Work out the finished part from the listing and answer in its coordinate system (mm). A direction names the side the tool comes from. Round coordinates to 2 decimals unless told otherwise and drop trailing zeros. Order: outer loops, then holes, each group sorted by start corner. A loop starts at its lowest first (then second) coordinate and runs counter-clockwise, first axis right, second up. Notation, with made-up numbers: (-13, 6) - (0, 6) arc R25 cw to (0, 40) - close; hole circle Ø3 at (-13.75, -10). An arc over 180 degrees is marked (long way). Use CSV: the item, a comma, the result in double quotes.
from build123d import *

# Parameters (mm, degrees)
SKETCH1_R                = 5
BOSS_EXTRUDE1_DEPTH      = 10
SKETCH2_R                = 4.5
BOSS_EXTRUDE2_DEPTH      = 12
BOSS_EXTRUDE2_DEPTH_BACK = 10
SKETCH3_R                = 5
BOSS_EXTRUDE3_DEPTH      = 10
SKETCH4_R                = 6
BOSS_EXTRUDE4_DEPTH      = 2
FILLET1_R                = 3


with BuildPart() as part:
    # Sketch1 → Boss-Extrude1 (new body)
    with BuildSketch(Plane(origin=(0, 0, 0), x_dir=(1, 0, 0), z_dir=(0, 1, 0))):
        with BuildLine():
            ThreePointArc((-10, 0), (0, -10), (10, 0))
            ThreePointArc((10, 0), (-47.75, 57.75), (-105.5, 0))
            ThreePointArc((-105.5, 0), (-95.5, -10), (-85.5, 0))
            ThreePointArc((-85.5, 0), (-47.75, 37.75), (-10, 0))
        make_face()
        with Locations((-95.5, 0)):
            Circle(SKETCH1_R, mode=Mode.SUBTRACT)
        Circle(SKETCH1_R, mode=Mode.SUBTRACT)
    extrude(amount=BOSS_EXTRUDE1_DEPTH)



with BuildPart() as body_2:
    # Sketch2 → Boss-Extrude2 (new body, two sides)
    with BuildSketch(Plane(origin=(0, 10, 0), x_dir=(1, 0, 0), z_dir=(0, 1, 0))) as boss_extrude2_sk:
        Circle(SKETCH2_R)
    extrude(amount=BOSS_EXTRUDE2_DEPTH)
    extrude(boss_extrude2_sk.sketch, amount=-BOSS_EXTRUDE2_DEPTH_BACK)


with BuildPart() as part_1:
    add(part.part)

    add(body_2.part)  # Boss-Extrude3 merges body 2
    # Sketch3 → Boss-Extrude3 (add)
    with BuildSketch(Plane(origin=(0, 10, 0), x_dir=(1, 0, 0), z_dir=(0, 1, 0))):
        Circle(SKETCH3_R)
    extrude(amount=-BOSS_EXTRUDE3_DEPTH)

    # Sketch4 → Boss-Extrude4 (add)
    with BuildSketch(Plane(origin=(0, 10, 0), x_dir=(1, 0, 0), z_dir=(0, 1, 0))):
        Circle(SKETCH4_R)
    extrude(amount=BOSS_EXTRUDE4_DEPTH)

    # Fillet1
    fillet1_edges = [part_1.edges().sort_by_distance(p)[0] for p in [
        (-47.75, 10, -37.75),
        (0, 10, 10),
        (-47.75, 10, -57.75),
        (0, 0, 10),
        (-47.75, 0, -37.75),
        (-95.5, 0, 10),
        (-47.75, 0, -57.75),
        (-95.5, 10, 10),
    ]]
    fillet(fillet1_edges, radius=FILLET1_R)


solid = part_1.part
(1) Find section B-B (x = -47.75). Determine the outline of the cut face in (y, z), and give its area (3 significant figures).
Findings below:
outline,"(0, -54.75) arc R3 ccw to (3, -57.75) - (7, -57.75) arc R3 ccw to (10, -54.75) - (10, -40.75) arc R3 ccw to (7, -37.75) - (3, -37.75) arc R3 ccw to (0, -40.75) - close"
area,"192 mm²"
(2) Find the intervals of material crossed by L1, parallel to X at y = 3.25, z = 0; L2, parallel to Y at x = -52.5, z = -41.5; L3, parallel to Z at x = -95.5, y = 4.5, in increasing order. Write a range as from..to.
Findings below:
L1,"x = -105.5..-100.5, -90.5..-85.5, -10..10"
L2,"y = 0..10"
L3,"z = -32.48..-5, 5..10"
(3) Find section C-C (y = 15.5). Determine the outline of the cut face in (x, z), and give its area (3 significant figures).
Findings below:
outline,"circle Ø9 at (0, 0)"
area,"63.6 mm²"
(4) Find section A-A (y = 4.25). Determine the outline of the cut face in (x, z).
Findings below:
outline,"(-105.5, 0) arc R57.75 ccw to (10, 0) arc R10 ccw to (-10, 0) arc R37.75 cw to (-85.5, 0) arc R10 ccw to start; hole circle Ø10 at (-95.5, 0)"
(5) The mould has two halves that part along X. Classify faces 3 (the cylindrical face through (-95.7, 5, 10)), 4 (the flat face through (-44, 0, -42)), 5 (the cylindrical face through (-0.59, 17.07, -4.46)): released by +X, released by -X, zero draft, split by the parting line, or undercut.
Findings below:
face 3,"undercut"
face 4,"zero draft"
face 5,"split by the parting line"
(6) For faces 1 (the flat face through (0, 22, 0)), 2 (the cylindrical face through (-6, 11, 0)), determine the directions among +Z, -Z, +X, -X, +Y, -Y from which every point of the face is accessible in a straight line to the end or side of a thin tool.
Findings below:
face 1,"+Z, -Z, +X, -X, +Y"
face 2,"+Y"
(7) Each of these flat-tipped pins is pushed along its axis until it touches: pin 1 (6 mm diameter, centred on x = -8.5, y = 12, fed in from -Z); pin 2 (8 mm diameter, centred on x = -95.5, z = 0, fed in from -Y). Where does it stop, or does it pass through?
Findings below:
pin 1,"stops at z = -42.11"
pin 2,"passes through"
